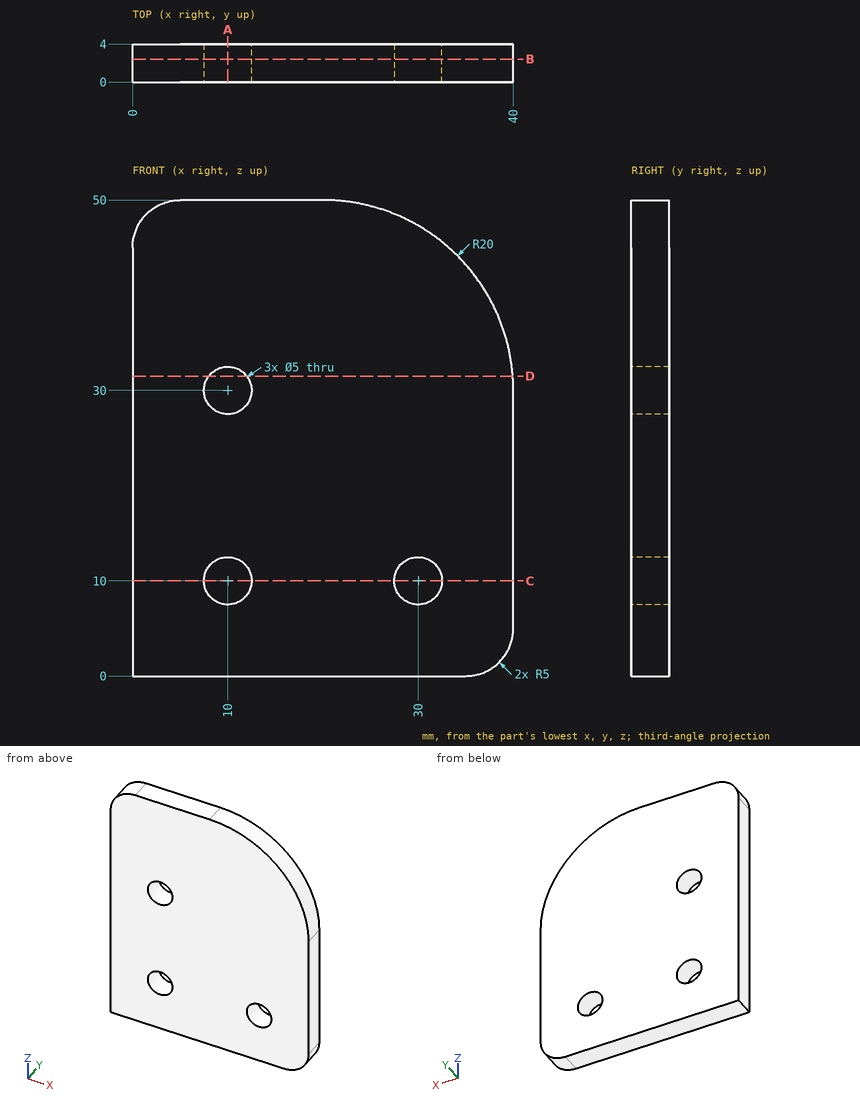
Input: dimensioned drawing with shaded views. Units: mm. Origin: part minimum x, y, z. Coordinates: 2 decimals unless noted, no trailing zeros. Order: outer loops, then holes, each group sorted by start corner. A loop starts at its lowest first (then second) coordinate and runs counter-clockwise, first axis right, second up. Notation, with made-up numbers: (-11, 54.5) - (27, 54.5) arc R17 cw to (27, 72.5) - close; hole circle Ø3 at (60, 63). An arc over 180 degrees is marked (long way). Return JSON: item names as keys, results as strings. Group by question number.
1. Cut plane C-C (z = 10). Output: boundary loops of the cut face in (x, y), plus the area to 3 significant figures.
2. Cut plane B-B (y = 2.4). Output: boundary loops of the cut face in (x, z).
3. Material intervals for line 1 along X through (y, z) = (2.45, 10); line 2 along Z through (x, y) = (10, 1.6); line 3 along X through (y, z) = (1.45, 30), sorted ascending. Write a range as [from, to].
4. Cut plane A-A (x = 10). Output: boundary loops of the cut face in (y, z).
5. Cut plane D-D (z = 31.5). Output: boundary loops of the cut face in (x, y), plus the area to 3 significant figures.
Resolved:
{
 "1": {"outline": "(0, 0) - (7.5, 0) - (7.5, 4) - (0, 4) - close; (12.5, 0) - (27.5, 0) - (27.5, 4) - (12.5, 4) - close; (32.5, 0) - (40, 0) - (40, 4) - (32.5, 4) - close", "area": "120 mm²"},
 "2": {"outline": "(0, 0) - (35, 0) arc R5 ccw to (40, 5) - (40, 30) arc R20 ccw to (20, 50) - (5, 50) arc R5 ccw to (0, 45) - close; hole circle Ø5 at (10, 10); hole circle Ø5 at (10, 30); hole circle Ø5 at (30, 10)"},
 "3": {"line 1": "x = [0, 7.5], [12.5, 27.5], [32.5, 40]", "line 2": "z = [0, 7.5], [12.5, 27.5], [32.5, 50]", "line 3": "x = [0, 7.5], [12.5, 40]"},
 "4": {"outline": "(0, 0) - (4, 0) - (4, 7.5) - (0, 7.5) - close; (0, 12.5) - (4, 12.5) - (4, 27.5) - (0, 27.5) - close; (0, 32.5) - (4, 32.5) - (4, 50) - (0, 50) - close"},
 "5": {"outline": "(0, 0) - (8, 0) - (8, 4) - (0, 4) - close; (12, 0) - (39.94, 0) - (39.94, 4) - (12, 4) - close", "area": "144 mm²"}
}
